Source: three-view drawing plus pictorial views. Frame: mm from the lowest corner of the part. Give positions to 0.01 mm unless a question says otherwise; leave off trailing zeros. Order: outer loops, then holes, each group sorted by start corner. A loop starts at its lowest first (then second) coordinate and runs counter-clockwise, first axis right, second up. Notation, with made-up numbers: (-25, 13) -> (30, 13) arc R35 ccw to (30, 52) -> close; hole circle Ø2 at (64.5, 80.25). An arc over 180 degrees is marked (long way). One line per question, with ' | ' between items.
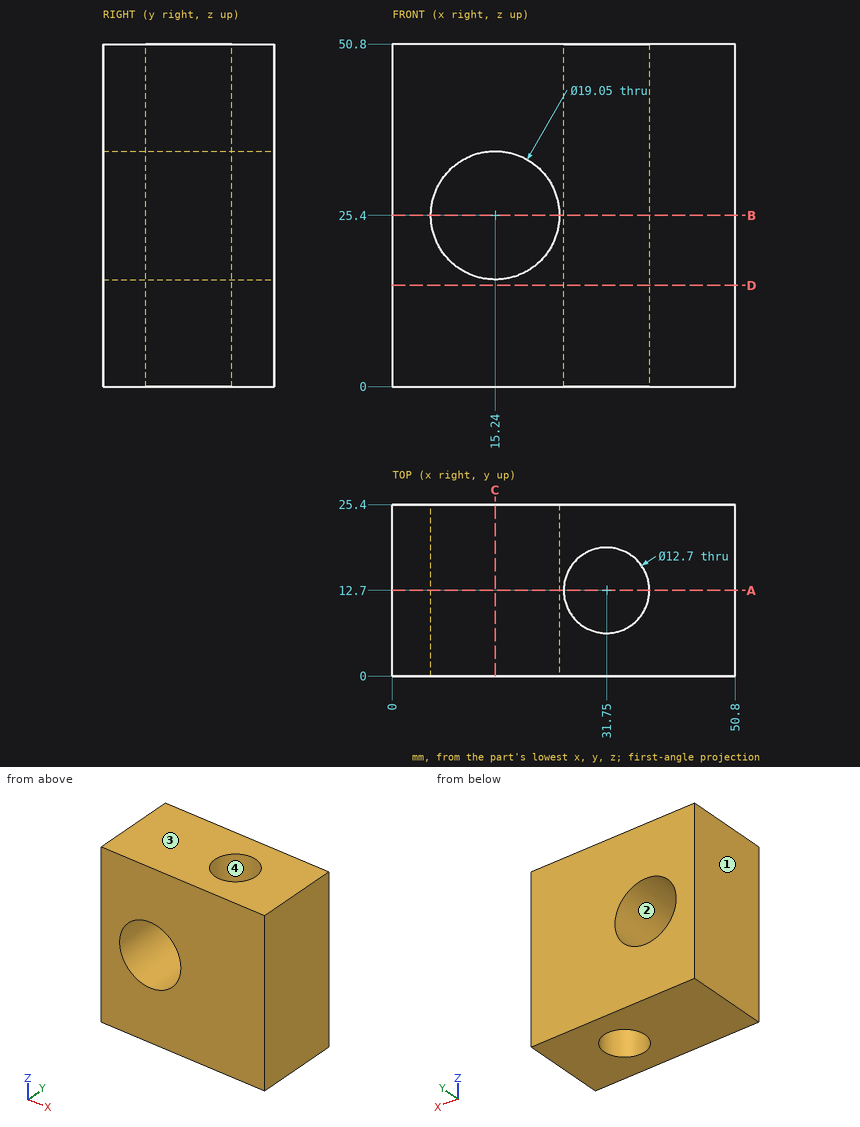
1) Material intervals for probe 1 along Y at (x, z) = (31.75, 17); probe 2 along Z at (x, y) = (15.24, 14.25) (3 decimals); probe 3 along X at (y, z) = (13, 25.4) (3 decimals), sorted ascending. Write a range as from..to.
Check result:
probe 1: y = 0..6.35, 19.05..25.4 | probe 2: z = 0..15.875, 34.925..50.8 | probe 3: x = 0..5.715, 24.765..25.407, 38.093..50.8
2) Section B-B on z = 25.4. Return loops of the section in (x, y) (3 decimals).
Check result:
outline: (0, 0) -> (5.715, 0) -> (5.715, 25.4) -> (0, 25.4) -> close; (24.765, 0) -> (50.8, 0) -> (50.8, 25.4) -> (24.765, 25.4) -> close; hole circle Ø12.7 at (31.75, 12.7)
3) Section C-C on x = 15.24. Return loops of the section in (y, z) (3 decimals).
Check result:
outline: (0, 0) -> (25.4, 0) -> (25.4, 15.875) -> (0, 15.875) -> close; (0, 34.925) -> (25.4, 34.925) -> (25.4, 50.8) -> (0, 50.8) -> close
4) Section A-A on y = 12.7. Return loops of the section in (x, z) (3 decimals), plus the area to 3 significant figures.
Check result:
outline: (0, 0) -> (25.4, 0) -> (25.4, 50.8) -> (0, 50.8) -> close; (38.1, 0) -> (50.8, 0) -> (50.8, 50.8) -> (38.1, 50.8) -> close; hole circle Ø19.05 at (15.24, 25.4) | area: 1,650 mm^2
5) Pull-direction query (X, two-part tool) for the marked faces 1, 2, 3 and 4; classes: +X half, -X half, draft (parallel to the pull), parting line (faces both ways), or undercut.
Check result:
face 1: -X half | face 2: undercut | face 3: draft | face 4: undercut
6) Section D-D on z = 15. Return loops of the section in (x, y).
Check result:
outline: (0, 0) -> (50.8, 0) -> (50.8, 25.4) -> (0, 25.4) -> close; hole circle Ø12.7 at (31.75, 12.7)
